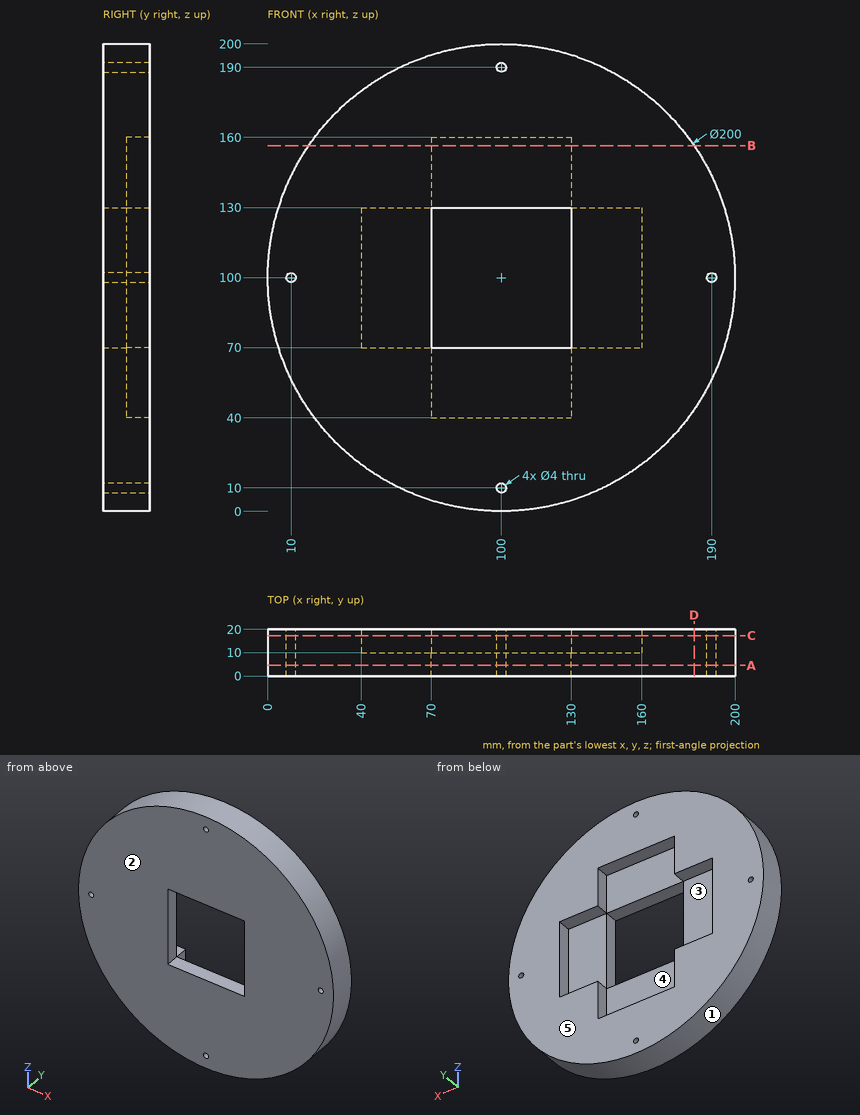
For this review, use the dimensioned drawing (mm, ordinates from the lowest corner) and the shaded views. A direction names the side the tool comes from. Round coordinates to 2 decimals unless told otherwise and drop trailing zeros. Order: outer loops, then holes, each group sorted by start corner. A loop starts at its lowest first (then second) coordinate and runs counter-clockwise, first axis right, second up. Notation, with made-up numbers: (44.25, 41) - (50.25, 41) arc R26 ccw to (50.25, 69) - close; hole circle Ø6 at (30, 16). An arc over 180 degrees is marked (long way). Use one line per item in the form item = value.
Q1. Add section B-B on z = 156.5. Give the boundary of the cut face in (x, y).
Response values:
outline = (17.49, 0) - (182.51, 0) - (182.51, 20) - (130, 20) - (130, 10) - (70, 10) - (70, 20) - (17.49, 20) - close
Q2. Add section D-D on x = 182.5. Give the boundary of the cut face in (y, z), then the cut area to 3 significant figures.
Response values:
outline = (0, 43.49) - (20, 43.49) - (20, 156.51) - (0, 156.51) - close
area = 2,260 mm^2
Q3. Mouldability with a two-part tool opening along Z and no side actions: class the marked faces 1, 2 and 3 as pulls with the +Z half, pulls with the -Z half, needs draft (parallel to the pull), parting line crosses it, or undercut.
Response values:
face_1 = parting line crosses it
face_2 = needs draft
face_3 = undercut
Q4. Tool access review of the marked faces 4 and 5: name each direction out of +Z, -Z, +X, -X, +Y, -Y from which nothing blocks a thin tool from reaching the whole face with its end or side.
Response values:
face_4 = +Y
face_5 = +Z, -Z, +X, -X, +Y
Q5. Clearance check with flat-ended pins moving along their axes: P1, Ø3, axis at x = 100, z = 190, coming from the +Y side; P2, Ø8, axis at x = 142, y = 13, coming from the -Z side; P3, Ø12, axis at y = 11.5, z = 112, coming from the +X side; P4, Ø3, axis at x = 55.5, y = 13.5, coming from the +Z side. State where each tip first meets the part, or that it passes through.
Response values:
P1 = through
P2 = 7.5
P3 = 199.82
P4 = 190.28
Q6. To check wall thickness, follow line 1 (X direction, y = 15.5, z = 100); line 2 (Y direction, x = 142, z = 82); line 3 (Z direction, x = 190, y = 11.5). State the ranges of each line that lie inside material, in increasing order.
Response values:
line_1 = 0 to 8, 12 to 40, 160 to 188, 192 to 200
line_2 = 0 to 10
line_3 = 56.41 to 98, 102 to 143.59
Q7. Add section C-C on y = 17.25. Give the boundary of the cut face in (x, z), then the cut area to 3 significant figures.
Response values:
outline = circle Ø200 at (100, 100); hole circle Ø4 at (10, 100); hole (40, 70) - (70, 70) - (70, 40) - (130, 40) - (130, 70) - (160, 70) - (160, 130) - (130, 130) - (130, 160) - (70, 160) - (70, 130) - (40, 130) - close; hole circle Ø4 at (100, 10); hole circle Ø4 at (100, 190); hole circle Ø4 at (190, 100)
area = 20,600 mm^2
Q8. Add section A-A on y = 4.5. Give the boundary of the cut face in (x, z).
Response values:
outline = circle Ø200 at (100, 100); hole circle Ø4 at (10, 100); hole (70, 70) - (130, 70) - (130, 130) - (70, 130) - close; hole circle Ø4 at (100, 10); hole circle Ø4 at (100, 190); hole circle Ø4 at (190, 100)
